Can you work these out from the model? Positions are in its coordinate system, mm. A direction names the side the tool comes from. Coordinates: 2 decimals unless noted, no trailing zeros. Order: outer loops, then holes, each group sorted by start corner. A loop starts at its lowest first (then second) coordinate and runs counter-clockwise, first axis right, second up.
```python
from build123d import *

# Parameters (mm, degrees)
SKETCH1_W           = 20.32
SKETCH1_H           = 20.32
BOSS_EXTRUDE1_DEPTH = 6.35
CUT_EXTRUDE1_DEPTH  = 5.08
SKETCH4_W           = 0.381
SKETCH4_H           = 21.648681081
CUT_EXTRUDE2_DEPTH  = 5.08


with BuildPart() as part:
    # Sketch1 → Boss-Extrude1 (new body)
    with BuildSketch(Plane(origin=(0, 0, 0), x_dir=(0, 1, 0), z_dir=(0, 0, 1))):
        with Locations((10.16, 10.16)):
            Rectangle(SKETCH1_W, SKETCH1_H)
    extrude(amount=BOSS_EXTRUDE1_DEPTH)

    # Sketch2 → Cut-Extrude1 (cut)
    with BuildSketch(Plane.XY.offset(6.35)):
        Polygon((-10.795, 18.415), (-8.255, 18.415), (-8.255, 20.32), (-4.445, 20.32), (-4.445, 18.415), (-1.905, 18.415), (-1.905, 1.905), (-4.445, 1.905), (-4.445, -0.532919187), (-8.255, -0.532919187), (-8.255, 1.905), (-10.795, 1.905), align=None)
    extrude(amount=-CUT_EXTRUDE1_DEPTH, mode=Mode.SUBTRACT)

    # Sketch4 → Cut-Extrude2 (cut)
    with BuildSketch(Plane.XY.offset(6.35)):
        with Locations((-18.8595, 9.956894273)):
            Rectangle(SKETCH4_W, SKETCH4_H)
        with Locations((-17.2085, 9.956894273)):
            Rectangle(SKETCH4_W, SKETCH4_H)
    extrude(amount=-CUT_EXTRUDE2_DEPTH, mode=Mode.SUBTRACT)


solid = part.part
```
1. Imagine slicing it at B-B on x = -8.5. Please give me the cut outline in (y, z) (3 decimals).
Completed:
outline: (0, 0) - (20.32, 0) - (20.32, 6.35) - (18.415, 6.35) - (18.415, 1.27) - (1.905, 1.27) - (1.905, 6.35) - (0, 6.35) - close
2. Please list where these lines run through material, in increasing order: probe 1 along X at (y, z) = (1, 2.5) (3 decimals); probe 2 along X at (y, z) = (15.75, 3) (3 decimals); probe 3 along Z at (x, y) = (-5.5, 2.25).
Completed:
probe 1: x = -20.32 to -19.05, -18.669 to -17.399, -17.018 to -8.255, -4.445 to 0
probe 2: x = -20.32 to -19.05, -18.669 to -17.399, -17.018 to -10.795, -1.905 to 0
probe 3: z = 0 to 1.27
3. Imagine slicing it at C-C on y = 8.5. Please give me the cut outline in (x, z) (3 decimals), then the cut area to 3 significant figures.
Completed:
outline: (-20.32, 0) - (0, 0) - (0, 6.35) - (-1.905, 6.35) - (-1.905, 1.27) - (-10.795, 1.27) - (-10.795, 6.35) - (-17.018, 6.35) - (-17.018, 1.27) - (-17.399, 1.27) - (-17.399, 6.35) - (-18.669, 6.35) - (-18.669, 1.27) - (-19.05, 1.27) - (-19.05, 6.35) - (-20.32, 6.35) - close
area: 80.0 mm2
4. On a 3-axis mill with a long thin cutter (end or side, diameter ignored), from which of +Z, -Z, +X, -X, +Y, -Y can I reach the whole of each face in a straight line? I mean faces 4 (the flat face through (-10, 1.905, 4)), 5 (the flat face through (-10, 20.32, 3)), 6 (the flat face through (-4.445, 19, 4)). Say none if no direction works.
Completed:
face 4: +Z
face 5: +Z, -Z, +X, -X, +Y
face 6: +Z, +Y, -Y
5. I'm going to push a flat-ended pin straight in: pin 1 (4.5 mm diameter, centred on x = -7.5, y = 9, fed in from +Z). Where does the tip first touch, or does it pass through?
Completed:
pin 1: stops at z = 1.27
6. Imagine slicing it at A-A on z = 2.75. Please give me the cut outline in (x, y) (3 decimals), then the cut area to 3 significant figures.
Completed:
outline: (-20.32, 0) - (-19.05, 0) - (-19.05, 20.32) - (-20.32, 20.32) - close; (-18.669, 0) - (-17.399, 0) - (-17.399, 20.32) - (-18.669, 20.32) - close; (-17.018, 0) - (-8.255, 0) - (-8.255, 1.905) - (-10.795, 1.905) - (-10.795, 18.415) - (-8.255, 18.415) - (-8.255, 20.32) - (-17.018, 20.32) - close; (-4.445, 0) - (0, 0) - (0, 20.32) - (-4.445, 20.32) - (-4.445, 18.415) - (-1.905, 18.415) - (-1.905, 1.905) - (-4.445, 1.905) - close
area: 236 mm2
7. Thinking about a two-plate mould opening in X: for faces 1 (the flat face through (-6, 10, 1.27)), 2 (the flat face through (-14, 10, 6.35)), 3 (the flat face through (-20.32, 10, 3)), which applies, pulls with the +X half, pulls with the -X half, needs draft (parallel to the pull), parting line crosses it, or undercut?
Completed:
face 1: undercut
face 2: needs draft
face 3: pulls with the -X half
